from build123d import *

# Parameters (mm, degrees)
F0_W     = 22.86
F0_H     = 83.82
F1_DEPTH = 48.26
F3_DEPTH = 19.05
F5_DEPTH = 22.86


with BuildPart() as f1:
    # F0 (on Top) → F1 (new body)
    with BuildSketch(Plane.XY):
        with Locations((11.43, 41.91)):
            Rectangle(F0_W, F0_H)
    extrude(amount=F1_DEPTH)

    # F2 (on face) → F3 (join)
    with BuildSketch(Plane(origin=(0, 83.82, 0), x_dir=(-1, 0, 0), z_dir=(0, 1, 0))):
        Polygon((-8.255, 40.005), (-11.43, 40.005), (-11.43, 36.83), (-11.43, 33.655), (-8.255, 33.655), align=None)
        Polygon((-8.255, 14.605), (-11.43, 14.605), (-14.605, 14.605), (-14.605, 8.255), (-8.255, 8.255), align=None)
        Polygon((-11.43, 36.83), (-11.43, 40.005), (-14.605, 40.005), (-14.605, 33.655), (-11.43, 33.655), align=None)
    extrude(amount=F3_DEPTH)

    # F4 (on Right) → F5 (join)
    with BuildSketch(Plane.YZ):
        Polygon((-35.780966, 0), (0, 0), (0, 48.468489), align=None)
    extrude(amount=F5_DEPTH)


solid = f1.part
Here's how the part is built. I have some questions about the finished solid (model axes, mm). A direction names the side the tool comes from. Give positions to 0.01 mm unless a question says otherwise; leave off trailing zeros. Write each loop counter-clockwise with the first axis right and the second up, starting at its lowest first coordinate (ties: lowest second). Pieces come first, ordered by that corner, then holes. Notation, with made-up numbers: (49.25, -13.5) -> (53.25, -13.5) arc R12 cw to (53.25, -8.5) -> close; hole circle Ø7 at (32.25, 37.5). An arc over 180 degrees is marked (long way). Use one line per item in the form item = value. Start each with the question number.
1. If I drill on L1, parallel to Z at x = 12.25, y = 88 (3 decimals); L2, parallel to Z at x = 15, y = 47; L3, parallel to Y at x = 2, z = 38, over which ranges is the centre line in solid material (lowest first)?
2. Imagine slicing it at C-C on z = 13. List the corners of the cut face in (x, y) for me (3 decimals).
3. Imagine slicing it at D-D on x = 10. List the corners of the cut face in (y, z) for me (3 decimals).
4. Imagine slicing it at B-B on x = 18.5. List the corners of the cut face in (y, z) for me, plus the area to 3 significant figures.
5. Will these pins go through, and if not, where does the flat tip stop? pin 1 Ø7 at (x, z) = (16.5, 20) entering from +Y; pin 2 Ø3 at (y, z) = (92.5, 11) entering from +X (3 decimals); pin 3 Ø5 at (x, y) = (11.5, 90) entering from +Z (3 decimals); pin 4 Ø3 at (x, y) = (9.5, 12) entering from -Z.
6. Imagine slicing it at A-A on y = 88. List the corners of the cut face in (x, z) for me (3 decimals), plus the area to 3 significant figures.
7. Thinking about a two-plate mould opening in Z: for faces 6 (the face through (14.605, 93, 11)), 7 (the face through (11, 42, 48.26)), 8 (the face through (11, 93, 14.605)), 9 (the face through (11, 93, 33.655)), which applies, +Z half, -Z half, draft (parallel to the pull), parting line (faces both ways), or undercut?
8. On a 3-axis mill with a long thin cutter (end or side, diameter ignored), from which of +Z, -Z, +X, -X, +Y, -Y can I reach the whole of each face in a straight line? I mean faces 1 (the face through (11.27, -17.64, 24.574)), 2 (the face through (11, 93, 40.005)), 3 (the face through (8.255, 93, 11)), 4 (the face through (14.605, 93, 37)), 5 (the face through (11, 93, 8.255)). Say none if no direction works.
Entries:
q1.L1 = 8.255 to 14.605, 33.655 to 40.005
q1.L2 = 0 to 48.26
q1.L3 = -7.73 to 83.82
q2.outline = (0, -26.184) -> (22.86, -26.184) -> (22.86, 83.82) -> (14.605, 83.82) -> (14.605, 102.87) -> (8.255, 102.87) -> (8.255, 83.82) -> (0, 83.82) -> close
q3.outline = (-35.781, 0) -> (83.82, 0) -> (83.82, 8.255) -> (102.87, 8.255) -> (102.87, 14.605) -> (83.82, 14.605) -> (83.82, 33.655) -> (102.87, 33.655) -> (102.87, 40.005) -> (83.82, 40.005) -> (83.82, 48.26) -> (0, 48.26) -> (0, 48.468) -> close
q4.outline = (-35.78, 0) -> (83.82, 0) -> (83.82, 48.26) -> (0, 48.26) -> (0, 48.47) -> close
q4.area = 4,910 mm²
q5.pin_1 = 83.82
q5.pin_2 = 14.605
q5.pin_3 = 40.005
q5.pin_4 = 0
q6.outline = (8.255, 8.255) -> (14.605, 8.255) -> (14.605, 14.605) -> (8.255, 14.605) -> close; (8.255, 33.655) -> (14.605, 33.655) -> (14.605, 40.005) -> (8.255, 40.005) -> close
q6.area = 80.6 mm²
q7.face_6 = draft
q7.face_7 = +Z half
q7.face_8 = undercut
q7.face_9 = undercut
q8.face_1 = +Z, +X, -X, -Y
q8.face_2 = +Z, +X, -X, +Y
q8.face_3 = +Z, -Z, -X, +Y
q8.face_4 = +Z, -Z, +X, +Y
q8.face_5 = -Z, +X, -X, +Y
